```python
from build123d import *

# Parameters (mm, degrees)
F1_DEPTH  = 3.125
F2_W      = 6
F2_H      = 50
F2_W_2    = 50
F2_H_2    = 6
F3_DEPTH  = 2
F4_R      = 2.6
F5_DEPTH  = 25
F6_W      = 6
F6_H      = 12.6
F6_H_2    = 15.2
F7_DEPTH  = 2
F8_W      = 12.6
F8_H      = 6
F8_W_2    = 15.2
F9_DEPTH  = 2
F10_R     = 2
F12_DEPTH = 25
F13_R     = 2


# Not quite as in the source:
# - a feature names something its author has since deleted; it is built from what else it names


with BuildPart() as f1:
    # F0 (on Top) → F1 (new body)
    with BuildSketch(Plane.XY):
        with BuildLine():
            Line((35, 35), (15, 35))
            ThreePointArc((15, 35), (-4.5539513718, 4.5539513718), (-35, -15))
            Line((-35, -15), (-35, -35))
            Line((-35, -35), (35, -35))
            Line((35, -35), (35, 35))
        make_face()
    extrude(amount=F1_DEPTH)

    # F2 (on face) → F3 (join)
    with BuildSketch(Plane(origin=(0, 0, 0), x_dir=(1, 0, 0), z_dir=(0, 0, -1))):
        with Locations((25, -10)):
            Rectangle(F2_W, F2_H)
        with Locations((-10, 25)):
            Rectangle(F2_W_2, F2_H_2)
    extrude(amount=F3_DEPTH)

    # F4 (on face) → F5 (cut)
    with BuildSketch(Plane(origin=(0, 0, -2), x_dir=(1, 0, 0), z_dir=(0, 0, -1))):
        with Locations((25, -15)):
            Circle(F4_R)
        with Locations((25, 10)):
            Circle(F4_R)
        with Locations((10, 25)):
            Circle(F4_R)
        with Locations((-15, 25)):
            Circle(F4_R)
    extrude(amount=-F5_DEPTH, mode=Mode.SUBTRACT)

    # F6 (on face) → F7 (cut)
    with BuildSketch(Plane(origin=(0, 0, -2), x_dir=(1, 0, 0), z_dir=(0, 0, -1))):
        with Locations((25, 8.7)):
            Rectangle(F6_W, F6_H)
        with Locations((25, -15)):
            Rectangle(F6_W, F6_H_2)
    extrude(amount=-F7_DEPTH, mode=Mode.SUBTRACT)

    # F8 (on face) → F9 (cut)
    with BuildSketch(Plane(origin=(0, 0, -2), x_dir=(1, 0, 0), z_dir=(0, 0, -1))):
        with Locations((8.7, 25)):
            Rectangle(F8_W, F8_H)
        with Locations((-15, 25)):
            Rectangle(F8_W_2, F8_H)
    extrude(amount=-F9_DEPTH, mode=Mode.SUBTRACT)

    # F10
    f10_edges = [f1.edges().sort_by_distance(p)[0] for p in [
        (35, 35, 1.5625),
        (15, 35, 1.5625),
        (-35, -15, 1.5625),
        (-35, -35, 1.5625),
        (35, -35, 1.5625),
    ]]
    fillet(f10_edges, radius=F10_R)

    # F11 (on Top) → F12 (cut)
    with BuildSketch(Plane.XY):
        with BuildLine():
            Line((15, -10.0502525317), (15, 20))
            ThreePointArc((15, 20), (9.1151461726, 10.9887424757), (2.2488038315, 2.7009436368))
            Line((2.2488038315, 2.7009436368), (15, -10.0502525317))
        make_face()
        with BuildLine():
            ThreePointArc((-2.7009436368, -2.2488038315), (-10.9887424757, -9.1151461726), (-20, -15))
            Line((-20, -15), (10.0502525317, -15))
            Line((10.0502525317, -15), (-2.7009436368, -2.2488038315))
        make_face()
    extrude(amount=F12_DEPTH, mode=Mode.SUBTRACT)

    # F13
    f13_edges = [f1.edges().sort_by_distance(p)[0] for p in [
        (15, 20, 1.5625),
        (-20, -15, 1.5625),
        (2.248804, 2.700944, 1.5625),
        (-2.700944, -2.248804, 1.5625),
        (10.050253, -15, 1.5625),
        (15, -10.050253, 1.5625),
    ]]
    fillet(f13_edges, radius=F13_R)


solid = f1.part
```
For this review, take the finished solid that the model builds, in its own axes (mm). A direction names the side the tool comes from. Coordinates: 2 decimals unless noted, no trailing zeros. Loops run counter-clockwise (first coordinate to the right, second up) from the corner with the lowest first, then second, coordinate; pieces in that order, holes last. Notation, with made-up numbers: (-7.5, 66) - (42.5, 66) arc R6 ccw to (42.5, 75) - close; hole circle Ø3 at (23, -2.5). An arc over 180 degrees is marked (long way). Use one line per item in the form item = value. Start each with the question number.
1) Take a section at C-C (x = -16). State the section outline as (y, z) points (3 decimals).
2) To check wall thickness, follow probe 1 along Y at (x, z) = (25, 1.25); probe 2 along X at (y, z) = (-25, 1.05); probe 3 along X at (y, z) = (-10, 1.6). State the ranges of each line that lie inside material, in increasing order. Write a range as from..to.
3) Take a section at B-B (y = -25). State the section outline as (x, z) points (3 decimals).
4) Draft analysis for pull direction Y (two halves, no side actions). For faces 4 (the face through (-13.6, -27.19, 1.54)), 5 (the face through (25, -2.4, -1)), 6 (the face through (25, 29, -2)), state which applies: released by +Y, released by -Y, zero draft, split by the parting line, or undercut.
5) For faces 1 (the face through (-7.4, -25, -1)), 2 (the face through (25, 22.6, -1)), 3 (the face through (-14.946, -13.552, 1.584)), list the 3-axis set-ups (+Z, -Z, +X, -X, +Y, -Y) from which the entire face can be reached by the end or side of a thin tool; tool diameter is ignored.
6) Take a section at D-D (y = 6.5). State the section outline as (x, z) points (3 decimals), plus the area to 3 significant figures.
7) Take a section at A-A (z = -0.8). State the section outline as (x, y) points.
8) For pin 1 (1 mm diameter, centred on x = -3.5, z = -1.5, fed in from +Y); pin 2 (2 mm diameter, centred on y = -26, z = -0.5, fed in from +X); pin 3 (1 mm diameter, centred on x = 23.5, z = -1, fed in from -Y); pin 4 (21 mm diameter, centred on x = -2, y = -2, fed in from -Z), all flat-tipped, find the tip position at first contact; note any pin that passes through.
From the geometry:
q1.outline = (-35, 0) - (-27.4, 0) - (-27.4, 3.125) - (-35, 3.125) - close; (-22.6, 0) - (-5.037, 0) - (-5.037, 3.125) - (-22.6, 3.125) - close
q2.probe_1 = -35..-12.6, -7.4..12.4, 17.6..35
q2.probe_2 = -35..-17.6, -12.4..7.4, 12.6..35
q2.probe_3 = -24.02..-12.21, 5.05..22.4, 27.6..35
q3.outline = (-35, -2) - (-22.6, -2) - (-22.6, 0) - (-17.6, 0) - (-17.6, 3.125) - (-35, 3.125) - close; (-12.4, 0) - (-7.4, 0) - (-7.4, -2) - (2.4, -2) - (2.4, 0) - (7.4, 0) - (7.4, 3.125) - (-12.4, 3.125) - close; (12.6, 0) - (35, 0) - (35, 3.125) - (12.6, 3.125) - close
q4.face_4 = undercut
q4.face_5 = released by -Y
q4.face_6 = zero draft
q5.face_1 = -Z, +Y, -Y
q5.face_2 = -Z, +X, -X
q5.face_3 = +Z, -Z
q6.outline = (-2.669, 0) - (5.594, 0) - (5.594, 3.125) - (-2.669, 3.125) - close; (15, 0) - (22, 0) - (22, -2) - (28, -2) - (28, 0) - (35, 0) - (35, 3.125) - (15, 3.125) - close
q6.area = 100 mm2
q7.outline = (-35, -28) - (-22.6, -28) - (-22.6, -22) - (-35, -22) - close; (-7.4, -28) - (2.4, -28) - (2.4, -22) - (-7.4, -22) - close; (22, -2.4) - (28, -2.4) - (28, 7.4) - (22, 7.4) - close; (22, 22.6) - (28, 22.6) - (28, 35) - (22, 35) - close
q8.pin_1 = -22
q8.pin_2 = 35
q8.pin_3 = -2.4
q8.pin_4 = 0
